Verification items for the finished model (mm, model axes). Face numbers are marked on the shaded views. Give positions to 0.01 mm unless a question says otherwise; leave off trailing zeros. Loops run counter-clockwise (first coordinate to the right, second up) from the corner with the lowest first, then second, coordinate; pieces in that order, holes last. Notation, with made-up numbers: M 78.5,19 L 89.5,19 A21 cw 89.5,51 Z; hole C 17.25,88.5 d6. An arc over 180 degrees is marked long. Use CSV: the item, a comma, the result in double quotes.
from build123d import *

# Parameters (mm, degrees)
EXTRUDE_1_DEPTH     = 2
EXTRUDE_2_DEPTH     = 4
SKETCH_3_R          = 1.6
SKETCH_3_W          = 7.7
SKETCH_3_H          = 2
SKETCH_3_W_2        = 4
SKETCH_3_H_2        = 10
CUT_EXTRUDE_1_DEPTH = 2.7
SKETCH_4_R          = 1.6
CUT_EXTRUDE_2_DEPTH = 5
CHAMFER_1_SIZE      = 2
SKETCH_5_W          = 2
SKETCH_5_H          = 12.69
CUT_EXTRUDE_3_DEPTH = 1.5
SKETCH_6_W          = 2
SKETCH_6_H          = 10
CUT_EXTRUDE_4_DEPTH = 0.8


with BuildPart() as part:
    # 草图1 → 凸台-拉伸1 (new body)
    with BuildSketch(Plane(origin=(0, 0, 0), x_dir=(1, 0, 0), z_dir=(0, 1, 0))):
        with BuildLine():
            Line((-24.955, -29.72), (28.955, -29.72))
            ThreePointArc((28.955, -29.72), (58.675, 0), (28.955, 29.72))
            Line((28.955, 29.72), (-24.955, 29.72))
            ThreePointArc((-24.955, 29.72), (-27.783427125, 28.548427125), (-28.955, 25.72))
            Line((-28.955, 25.72), (-28.955, -25.72))
            ThreePointArc((-28.955, -25.72), (-27.783427125, -28.548427125), (-24.955, -29.72))
        make_face()
    extrude(amount=EXTRUDE_1_DEPTH)

    # 草图2 → 凸台-拉伸2 (add)
    with BuildSketch(Plane(origin=(0, 2, 0), x_dir=(1, 0, 0), z_dir=(0, 1, 0))):
        with BuildLine():
            Line((28.955, 29.72), (-24.955, 29.72))
            ThreePointArc((-24.955, 29.72), (-27.783427125, 28.548427125), (-28.955, 25.72))
            Line((-28.955, 25.72), (-28.955, -25.72))
            ThreePointArc((-28.955, -25.72), (-27.783427125, -28.548427125), (-24.955, -29.72))
            Line((-24.955, -29.72), (28.955, -29.72))
            ThreePointArc((28.955, -29.72), (58.675, 0), (28.955, 29.72))
        make_face()
        with BuildLine():
            Line((-26.955, 24.15458435), (-26.955, -24.15458435))
            ThreePointArc((-26.955, -24.15458435), (-23.8332124, -24.577957377), (-23.604365952, -27.72))
            Line((-23.604365952, -27.72), (28.955, -27.72))
            ThreePointArc((28.955, -27.72), (56.675, 0), (28.955, 27.72))
            Line((28.955, 27.72), (-23.604365952, 27.72))
            ThreePointArc((-23.604365952, 27.72), (-23.8332124, 24.577957377), (-26.955, 24.15458435))
        make_face(mode=Mode.SUBTRACT)
    extrude(amount=EXTRUDE_2_DEPTH)

    # 草图3 → 切除-拉伸1 (cut)
    with BuildSketch(Plane(origin=(0, 6, 0), x_dir=(1, 0, 0), z_dir=(0, 1, 0))):
        with Locations(Location((-25.655, 26.29, 0), (0, 0, 270))):
            Circle(SKETCH_3_R)
        with Locations(Location((-25.655, -26.29, 0), (0, 0, 270))):
            Circle(SKETCH_3_R)
        with Locations((-14.605, 28.72)):
            Rectangle(SKETCH_3_W, SKETCH_3_H)
        with Locations((-28.955, 0)):
            Rectangle(SKETCH_3_W_2, SKETCH_3_H_2)
    extrude(amount=-CUT_EXTRUDE_1_DEPTH, mode=Mode.SUBTRACT)

    # 草图4 → 切除-拉伸2 (cut)
    with BuildSketch(Plane(origin=(0, 6, 0), x_dir=(1, 0, 0), z_dir=(0, 1, 0))):
        with Locations(Location((-25.655, 26.29, 0), (0, 0, 270))):
            Circle(SKETCH_4_R)
        with Locations(Location((-25.655, -26.29, 0), (0, 0, 270))):
            Circle(SKETCH_4_R)
    extrude(amount=-CUT_EXTRUDE_2_DEPTH, mode=Mode.SUBTRACT)

    # 倒角1
    chamfer_1_edges = [part.edges().sort_by_distance(p)[0] for p in [
        (2, 0, 29.72),
        (-27.783427125, 0, 28.548427125),
        (-28.955, 0, 0),
        (-27.783427125, 0, -28.548427125),
        (2, 0, -29.72),
        (58.675, 0, 0),
    ]]
    chamfer(chamfer_1_edges, length=CHAMFER_1_SIZE)

    # 草图5 → 切除-拉伸3 (cut)
    with BuildSketch(Plane(origin=(0, 6, 0), x_dir=(1, 0, 0), z_dir=(0, 1, 0))):
        with Locations((-27.955, 16.635)):
            Rectangle(SKETCH_5_W, SKETCH_5_H)
    extrude(amount=-CUT_EXTRUDE_3_DEPTH, mode=Mode.SUBTRACT)

    # 草图6 → 切除-拉伸4 (cut)
    with BuildSketch(Plane(origin=(0, 3.3, 0), x_dir=(1, 0, 0), z_dir=(0, 1, 0))):
        with Locations((-27.955, 0)):
            Rectangle(SKETCH_6_W, SKETCH_6_H)
    extrude(amount=-CUT_EXTRUDE_4_DEPTH, mode=Mode.SUBTRACT)


solid = part.part
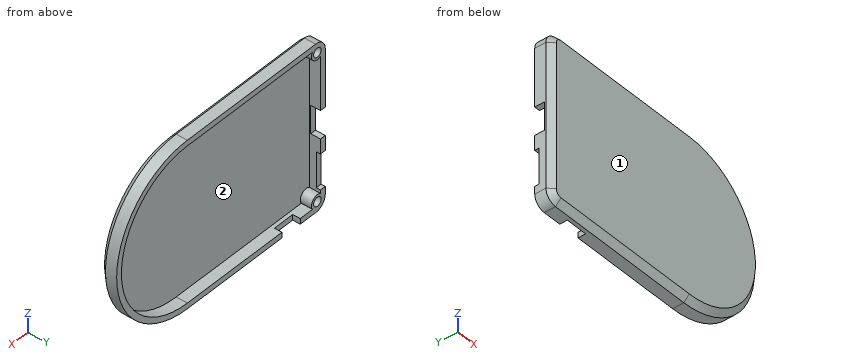
(1) Mould release check, pull along Z, two halves, no side actions. Record for the marked faces 1 and 2: released by +Z, released by -Z, zero draft, split by the parting line, or undercut.
Calculated:
face 1,"zero draft"
face 2,"undercut"
(2) Section check A-A on z = 0. Record the cut outline in (x, y) (3 decimals).
Calculated:
outline,"M -28.955,2 L -26.955,0 L 56.675,0 L 58.675,2 L 58.675,6 L 56.675,6 L 56.675,2 L -26.955,2 L -26.955,2.5 L -28.955,2.5 Z"
(3) Depth check by flat-ended pin: pin 1 Ø16.5 at (x, z) = (29.5, 13) entering from +Y; pin 2 Ø0.8 at (x, y) = (-27.5, 5.5) entering from -Z; pin 3 Ø2.5 at (x, z) = (-25.655, -26.29) entering from +Y; pin 4 Ø1.6 at (x, z) = (-26.5, 25.5) entering from +Y. Enter the tip coordinate at first touch or a pass-through.
Calculated:
pin 1,"stops at y = 2"
pin 2,"stops at z = -29.1"
pin 3,"stops at y = 1"
pin 4,"stops at y = 6"
(4) Scan lines: L1, parallel to Z at x = -5.5, y = 5; L2, parallel to X at y = 5.75, z = 16 (3 decimals); L3, parallel to Y at x = -11, z = 14. Record each from-to range of solid material in increasing order. Write a range as from..to.
Calculated:
L1,"z = -29.72..-27.72, 27.72..29.72"
L2,"x = -28.955..-26.955, 51.591..54.001"
L3,"y = 0..2"
